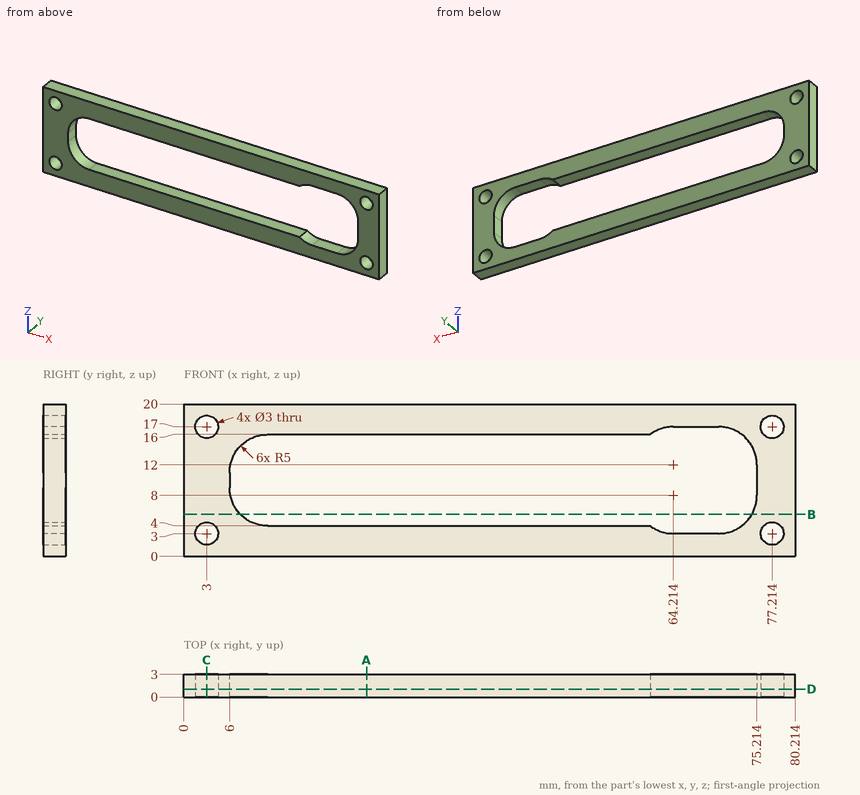
Here's the drawing with two shaded views (mm, measured from the low corner). I have some questions. Coordinates: 2 decimals unless noted, no trailing zeros. Write each loop counter-clockwise with the first axis right and the second up, starting at its lowest first coordinate (ties: lowest second). Pieces come first, ordered by that corner, then holes. Notation, with made-up numbers: (68.25, 81.25) - (106.25, 81.25) arc R23 ccw to (106.25, 100.25) - close; hole circle Ø11 at (73, -11). An arc over 180 degrees is marked (long way). Return JSON: item names as keys, results as strings.
Q1. If we section it at B-B (z = 5.5): Please give me the cut outline in (x, y).
Computed values:
{"outline": "(0, 0) - (7.43, 0) - (7.43, 3) - (0, 3) - close; (74.54, 0) - (80.21, 0) - (80.21, 3) - (74.54, 3) - close"}
Q2. Please list where these lines run through material, in increasing order: L1, parallel to Z at x = 61, y = 1.25; L2, parallel to X at y = 2.45, z = 17.5; L3, parallel to Z at x = 64.5, y = 1.9. Write a range as from..to.
Computed values:
{"L1": "z = 0..4, 16..20", "L2": "x = 0..1.59, 4.41..75.8, 78.63..80.21", "L3": "z = 0..3, 17..20"}
Q3. If we section it at A-A (x = 24): Please give me the cut outline in (y, z).
Computed values:
{"outline": "(0, 0) - (3, 0) - (3, 4) - (0, 4) - close; (0, 16) - (3, 16) - (3, 20) - (0, 20) - close"}
Q4. If we section it at D-D (y = 1.05): Please give me the cut outline in (x, z), then the cut area to 3 significant figures.
Computed values:
{"outline": "(0, 0) - (80.21, 0) - (80.21, 20) - (0, 20) - close; hole circle Ø3 at (3, 3); hole circle Ø3 at (3, 17); hole (6, 9) arc R5 ccw to (11, 4) - (61.21, 4) arc R5 ccw to (64.21, 3) - (70.21, 3) arc R5 ccw to (75.21, 8) - (75.21, 12) arc R5 ccw to (70.21, 17) - (64.21, 17) arc R5 ccw to (61.21, 16) - (11, 16) arc R5 ccw to (6, 11) - close; hole circle Ø3 at (77.21, 3); hole circle Ø3 at (77.21, 17)", "area": "741 mm2"}
Q5. If we section it at C-C (x = 3): Please give me the cut outline in (y, z), then the cut area to 3 significant figures.
Computed values:
{"outline": "(0, 0) - (3, 0) - (3, 1.5) - (0, 1.5) - close; (0, 4.5) - (3, 4.5) - (3, 15.5) - (0, 15.5) - close; (0, 18.5) - (3, 18.5) - (3, 20) - (0, 20) - close", "area": "42.0 mm2"}
